Geometry: final body of the model. Coordinates: model frame, mm. Coordinates: 2 decimals unless noted, no trailing zeros. Order: outer loops, then holes, each group sorted by start corner. A loop starts at its lowest first (then second) coordinate and runs counter-clockwise, first axis right, second up. Notation, with made-up numbers: (22.25, 45.5) - (30.25, 45.5) arc R12 cw to (30.25, 58.5) - close; hole circle Ø11 at (22.25, 84). An arc over 180 degrees is marked (long way). Use a Markdown table: item, result. Add a question column.
```python
from build123d import *

# Parameters (mm, degrees)
SKETCH_1_R          = 7.5
SKETCH_1_R_2        = 2.5
EXTRUDE_1_DEPTH     = 3
SKETCH_2_R          = 1.25
CUT_EXTRUDE_1_DEPTH = 10
CHAMFER_1_SIZE      = 1


with BuildPart() as part:
    # 草图1 → 凸台-拉伸1 (new body)
    with BuildSketch(Plane.XY):
        Circle(SKETCH_1_R)
        Circle(SKETCH_1_R_2, mode=Mode.SUBTRACT)
    extrude(amount=EXTRUDE_1_DEPTH)

    # 草图2 → 切除-拉伸1 (cut)
    with BuildSketch(Plane.XY.offset(3)):
        with Locations((0, 4.5)):
            Circle(SKETCH_2_R)
        with Locations((4.5, 0)):
            Circle(SKETCH_2_R)
        with Locations((0, -4.5)):
            Circle(SKETCH_2_R)
        with Locations((-4.5, 0)):
            Circle(SKETCH_2_R)
    extrude(amount=-CUT_EXTRUDE_1_DEPTH, mode=Mode.SUBTRACT)

    # 倒角1
    # the kernel refuses this chamfer: 1 mm, written as the material it takes off along each edge
    with BuildSketch(Plane(origin=(0, 4.5, 0), x_dir=(1, 0, 0), z_dir=(0, -1, 0))) as chamfer_1_piece_1:
        Polygon((1.25 + CHAMFER_1_SIZE, 0), (1.25, CHAMFER_1_SIZE), (1.25, 0), align=None)
    revolve(axis=Axis((0, 4.5, 0), (0, 0, 1)), mode=Mode.SUBTRACT)
    with BuildSketch(Plane(origin=(4.5, 0, 0), x_dir=(1, 0, 0), z_dir=(0, -1, 0))) as chamfer_1_piece_2:
        Polygon((1.25 + CHAMFER_1_SIZE, 0), (1.25, CHAMFER_1_SIZE), (1.25, 0), align=None)
    revolve(axis=Axis((4.5, 0, 0), (0, 0, 1)), mode=Mode.SUBTRACT)
    with BuildSketch(Plane(origin=(0, -4.5, 0), x_dir=(1, 0, 0), z_dir=(0, -1, 0))) as chamfer_1_piece_3:
        Polygon((1.25 + CHAMFER_1_SIZE, 0), (1.25, CHAMFER_1_SIZE), (1.25, 0), align=None)
    revolve(axis=Axis((0, -4.5, 0), (0, 0, 1)), mode=Mode.SUBTRACT)
    with BuildSketch(Plane(origin=(-4.5, 0, 0), x_dir=(1, 0, 0), z_dir=(0, -1, 0))) as chamfer_1_piece_4:
        Polygon((1.25 + CHAMFER_1_SIZE, 0), (1.25, CHAMFER_1_SIZE), (1.25, 0), align=None)
    revolve(axis=Axis((-4.5, 0, 0), (0, 0, 1)), mode=Mode.SUBTRACT)


solid = part.part
```
1) Section A-A (y = 0). Return loops of the section in (x, z), then the cut area to 3 significant figures.
2) Draft query along X for faces 1 (the face through (-7.493, 0.33, 1.479)), 2 (the face through (-0.27, 3.28, 2.01)), 3 (the face through (-2, 2, 0)). Return one class per face: pulls with the +X half, pulls with the -X half, needs draft (parallel to the pull), parting line crosses it, or undercut.
3) Section B-B (x = 4.5). Return loops of the section in (y, z).
4) Pin query (flat end, axial travel): pin 1 (1 mm diameter, centred on y = -5, z = 1.5, fed in from +X). Return the tip coordinate at first contact, or that it passes through.
5) Ray query, line 1 along Y through (x, z) = (0, 1.7); line 2 along Y through (x, z) = (1, 2.65); line 3 along Y through (x, z) = (1.5, 1.2). Return the intervals inside material, ascending.
6) Section D-D (z = 2.25). Return loops of the section in (x, y).
Values follow:
| question | item | result |
|---|---|---|
| 1 | outline | (-7.5, 0) - (-6.75, 0) - (-5.75, 1) - (-5.75, 3) - (-7.5, 3) - close; (-3.25, 1) - (-2.5, 0.25) - (-2.5, 3) - (-3.25, 3) - close; (2.5, 0.25) - (3.25, 1) - (3.25, 3) - (2.5, 3) - close; (5.75, 1) - (6.75, 0) - (7.5, 0) - (7.5, 3) - (5.75, 3) - close |
| 1 | area | 13.1 mm² |
| 2 | face 1 | parting line crosses it |
| 2 | face 2 | undercut |
| 2 | face 3 | needs draft |
| 3 | outline | (-6, 0) - (-2.25, 0) - (-1.25, 1) - (-1.25, 3) - (-6, 3) - close; (1.25, 1) - (2.25, 0) - (6, 0) - (6, 3) - (1.25, 3) - close |
| 4 | pin 1 | stops at x = 6 |
| 5 | line 1 | y = -7.5 to -5.75, -3.25 to -2.5, 2.5 to 3.25, 5.75 to 7.5 |
| 5 | line 2 | y = -7.43 to -5.25, -3.75 to -2.29, 2.29 to 3.75, 5.25 to 7.43 |
| 5 | line 3 | y = -7.35 to -2, 2 to 7.35 |
| 6 | outline | circle Ø15 at (0, 0); hole circle Ø2.5 at (-4.5, 0); hole circle Ø5 at (0, 0); hole circle Ø2.5 at (0, -4.5); hole circle Ø2.5 at (0, 4.5); hole circle Ø2.5 at (4.5, 0) |
